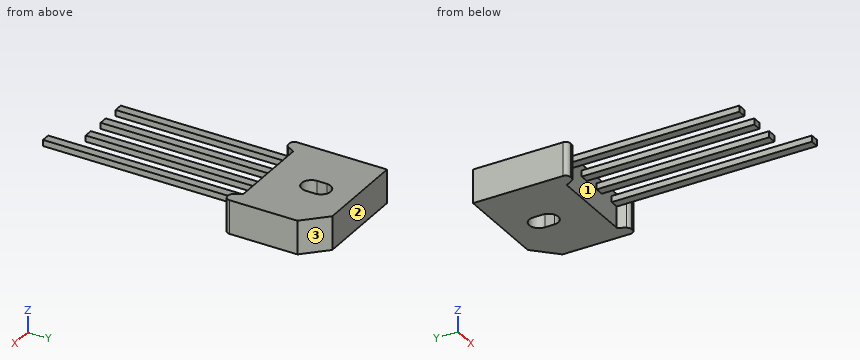
from build123d import *

# Parameters (mm, degrees)
BOSS_EXTRUDE1_DEPTH = 3.425
SKETCH2_W           = 1.75
SKETCH2_H           = 1.25
BOSS_EXTRUDE2_DEPTH = 35.15
SKETCH3_W           = 1.75
SKETCH3_H           = 1.25
BOSS_EXTRUDE3_DEPTH = 5.65


with BuildPart() as part:
    # Sketch1 → Boss-Extrude1 (new, symmetric)
    with BuildSketch(Plane.XY):
        with BuildLine():
            Line((7.15, 14.403910503), (-11.6, 14.403910503))
            Line((-11.6, 14.403910503), (-11.6, -2.896089497))
            Line((-11.6, -2.896089497), (-11.6, -3.896089497))
            ThreePointArc((-11.6, -3.896089497), (-11.307106781, -4.603196278), (-10.6, -4.896089497))
            Line((-10.6, -4.896089497), (-10.28914747, -4.896089497))
            ThreePointArc((-10.28914747, -4.896089497), (-9.78914747, -4.762114901), (-9.423122066, -4.396089497))
            Line((-9.423122066, -4.396089497), (-8.558813185, -2.899062602))
            Line((-8.558813185, -2.899062602), (8.558813185, -2.899062602))
            Line((8.558813185, -2.899062602), (9.423122066, -4.396089497))
            ThreePointArc((9.423122066, -4.396089497), (9.78914747, -4.762114901), (10.28914747, -4.896089497))
            Line((10.28914747, -4.896089497), (10.6, -4.896089497))
            ThreePointArc((10.6, -4.896089497), (11.307106781, -4.603196278), (11.6, -3.896089497))
            Line((11.6, -3.896089497), (11.6, -2.896089497))
            Line((11.6, -2.896089497), (11.6, 9.953910503))
            Line((11.6, 9.953910503), (7.15, 14.403910503))
        make_face()
        with BuildLine():
            ThreePointArc((-1.975, 7.853910503), (0, 9.828910503), (1.975, 7.853910503))
            Line((1.975, 7.853910503), (1.975, 5.903910503))
            ThreePointArc((1.975, 5.903910503), (0, 3.928910503), (-1.975, 5.903910503))
            Line((-1.975, 5.903910503), (-1.975, 7.853910503))
        make_face(mode=Mode.SUBTRACT)
    extrude(amount=BOSS_EXTRUDE1_DEPTH, both=True)

    # Sketch2 → Boss-Extrude2 (add)
    with BuildSketch(Plane.XZ.offset(2.899062602)):
        with Locations((-7.683813185, 1.525)):
            Rectangle(SKETCH2_W, SKETCH2_H)
        with Locations((-2.561271062, 1.525)):
            Rectangle(SKETCH2_W, SKETCH2_H)
        with Locations((2.561271062, 1.525)):
            Rectangle(SKETCH2_W, SKETCH2_H)
        with Locations((7.683813185, 1.525)):
            Rectangle(SKETCH2_W, SKETCH2_H)
    extrude(amount=BOSS_EXTRUDE2_DEPTH)

    # Sketch3 → Boss-Extrude3 (add)
    with BuildSketch(Plane.XZ.offset(38.049062602)):
        with Locations((7.683813185, 1.525)):
            Rectangle(SKETCH3_W, SKETCH3_H)
    extrude(amount=BOSS_EXTRUDE3_DEPTH)


solid = part.part
Here's how the part is built. I have some questions about the finished solid (model axes, mm). Face numbers are marked on the shaded views. Round coordinates to 2 decimals unless told otherwise and drop trailing zeros. Write each loop counter-clockwise with the first axis right and the second up, starting at its lowest first coordinate (ties: lowest second). Pieces come first, ordered by that corner, then holes. Notation, with made-up numbers: (78.5, -17) -> (83.5, -17) arc R8 cw to (83.5, -2) -> close; hole circle Ø7 at (9, 1). An arc over 180 degrees is marked (long way). One line per item, written item: value.
1) Suppose I cut it at D-D on x = -2.5. List the corners of the cut face in (y, z) for me (3 decimals).
Filled sheet:
outline: (-38.049, 0.9) -> (-2.899, 0.9) -> (-2.899, -3.425) -> (14.404, -3.425) -> (14.404, 3.425) -> (-2.899, 3.425) -> (-2.899, 2.15) -> (-38.049, 2.15) -> close
2) If I drill on line 1 (X direction, y = -18, z = 2); line 2 (Y direction, x = -5, z = -0.75); line 3 (Y direction, x = -10.25, z = 3), over which ranges is the centre line in solid material (lowest first)? Write a range as [from, to].
Filled sheet:
line 1: x = [-8.56, -6.81], [-3.44, -1.69], [1.69, 3.44], [6.81, 8.56]
line 2: y = [-2.9, 14.4]
line 3: y = [-4.9, 14.4]
3) Suppose I cut it at C-C on z = 0.25. List the corners of the cut face in (x, y) for me (3 decimals), plus the area to 3 significant figures.
Filled sheet:
outline: (-11.6, -3.896) arc R1 ccw to (-10.6, -4.896) -> (-10.289, -4.896) arc R1 ccw to (-9.423, -4.396) -> (-8.559, -2.899) -> (8.559, -2.899) -> (9.423, -4.396) arc R1 ccw to (10.289, -4.896) -> (10.6, -4.896) arc R1 ccw to (11.6, -3.896) -> (11.6, 9.954) -> (7.15, 14.404) -> (-11.6, 14.404) -> close; hole (-1.975, 5.904) arc R1.975 ccw to (1.975, 5.904) -> (1.975, 7.854) arc R1.975 ccw to (-1.975, 7.854) -> close
area: 381 mm2
4) Suppose I cut it at B-B on x = 0. List the corners of the cut face in (y, z) for me (3 decimals).
Filled sheet:
outline: (-2.899, -3.425) -> (3.929, -3.425) -> (3.929, 3.425) -> (-2.899, 3.425) -> close; (9.829, -3.425) -> (14.404, -3.425) -> (14.404, 3.425) -> (9.829, 3.425) -> close
5) I'm going to push flat-ended pins straight in: pin 1 Ø1.4 at (x, z) = (-7.5, 1.5) entering from -Y; pin 2 Ø0.5 at (x, y) = (-2, -13.5) entering from +Z; pin 3 Ø1 at (y, z) = (-24, 1) entering from +X. Where does each tip first touch, or does it pass through?
Filled sheet:
pin 1: stops at y = -38.05
pin 2: stops at z = 2.15
pin 3: stops at x = 8.56
6) We'd pull the mould along X, two halves only. Please class the marked faces 1, 2 and 3: released by +X, released by -X, zero draft, split by the parting line, or undercut.
Filled sheet:
face 1: undercut
face 2: zero draft
face 3: released by +X
7) Suppose I cut it at A-A on y = -23.5. List the corners of the cut face in (x, z) for me, plus the area to 3 significant figures.
Filled sheet:
outline: (-8.56, 0.9) -> (-6.81, 0.9) -> (-6.81, 2.15) -> (-8.56, 2.15) -> close; (-3.44, 0.9) -> (-1.69, 0.9) -> (-1.69, 2.15) -> (-3.44, 2.15) -> close; (1.69, 0.9) -> (3.44, 0.9) -> (3.44, 2.15) -> (1.69, 2.15) -> close; (6.81, 0.9) -> (8.56, 0.9) -> (8.56, 2.15) -> (6.81, 2.15) -> close
area: 8.75 mm2
